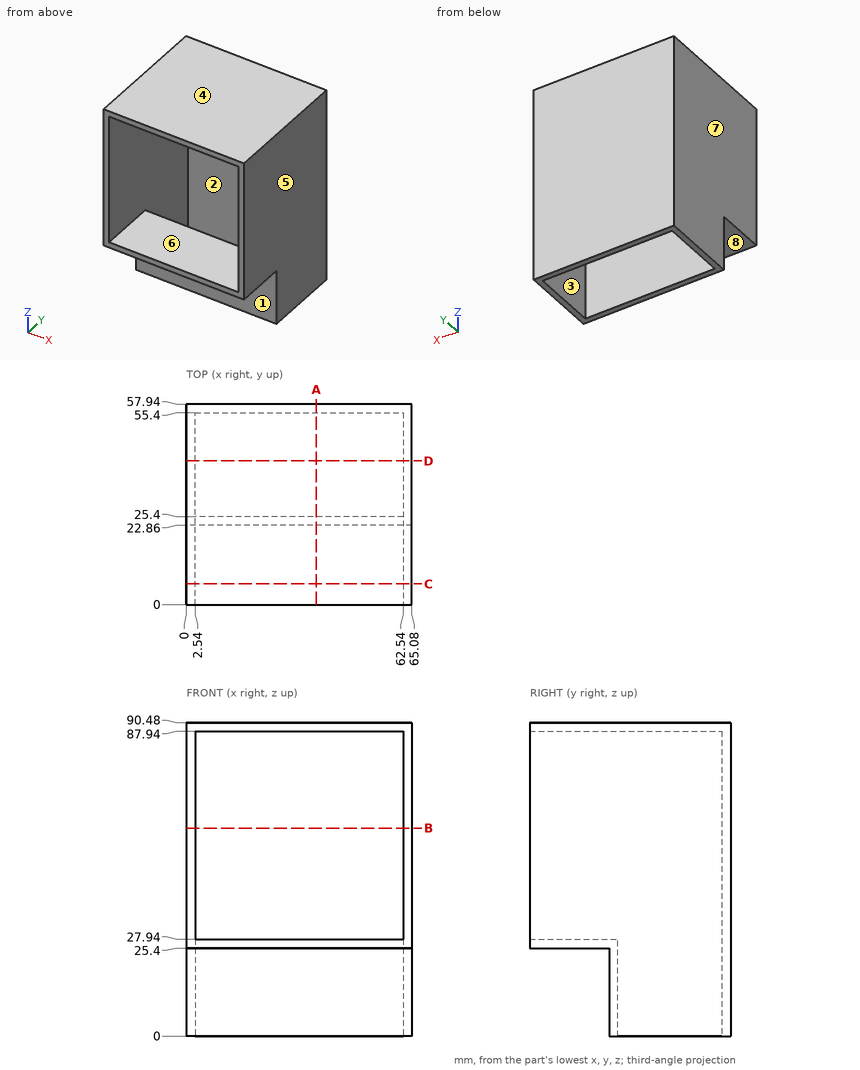
Job drawing, mm, ordinate dimensions from the low corner. One solid piece. A direction names the side the tool comes from. Coordinates: 2 decimals unless noted, no trailing zeros. Write each loop counter-clockwise with the first axis right and the second up, starting at its lowest first coordinate (ties: lowest second). Pieces come first, ordered by that corner, then holes. Notation, with made-up numbers: M -32,15.5 L 18,15.5 A24 ccw 18,49.5 Z; hole C 51.25,21 d6. An arc over 180 degrees is marked long. Answer as a JSON object with one key per item and string values. Group by question number.
1) Wall check: line 1 (X direction, y = 27, z = 41.5); line 2 (Y direction, x = 48.5, z = 5.5); line 3 (Z direction, x = 47.5, y = 8). Give the ranges that are in metal, low to high. Write a range as from..to.
2) Saw through at A-A (x = 37.5). Write the cut outline in (y, z), plus the area to 3 significant figures.
3) Saw through at C-C (y = 6). Write the cut outline in (x, z), plus the area to 3 significant figures.
4) Mould opens along X. For the marked faces 6, 7 and 8 say: +X half, -X half, draft (parallel to the pull), parting line (faces both ways), or undercut.
5) Saw through at B-B (z = 60). Write the cut outline in (x, y).
6) Saw through at D-D (y = 41.5). Write the cut outline in (x, z), plus the area to 3 significant figures.
7) Pin check, flat tips, straight feed: pin 1 Ø3 at (x, y) = (21, 36) entering from -Z; pin 2 Ø12.5 at (x, z) = (28, 7.5) entering from -Y; pin 3 Ø7 at (x, y) = (36, 9.5) entering from -Z; pin 4 Ø18 at (x, z) = (17.5, 23.5) entering from -Y. Stop position of each tip, or through.
8) Tool access for the marked faces 1, 2, 3, 4 and 5: list every direction of +Z, -Z, +X, -X, +Y, -Y with a clear straight run to the whole face (end or side of a thin tool).
Values follow:
{
 "1": {"line 1": "x = 0..2.54, 62.54..65.08", "line 2": "y = 22.86..25.4, 55.4..57.94", "line 3": "z = 25.4..27.94, 87.94..90.48"},
 "2": {"outline": "M 0,25.4 L 22.86,25.4 L 22.86,0 L 25.4,0 L 25.4,27.94 L 0,27.94 Z; M 0,87.94 L 55.4,87.94 L 55.4,0 L 57.94,0 L 57.94,90.48 L 0,90.48 Z", "area": "500 mm2"},
 "3": {"outline": "M 0,25.4 L 65.08,25.4 L 65.08,90.48 L 0,90.48 Z; hole M 2.54,27.94 L 62.54,27.94 L 62.54,87.94 L 2.54,87.94 Z", "area": "635 mm2"},
 "4": {"face 6": "undercut", "face 7": "-X half", "face 8": "draft"},
 "5": {"outline": "M 0,0 L 2.54,0 L 2.54,55.4 L 62.54,55.4 L 62.54,0 L 65.08,0 L 65.08,57.94 L 0,57.94 Z"},
 "6": {"outline": "M 0,0 L 2.54,0 L 2.54,87.94 L 62.54,87.94 L 62.54,0 L 65.08,0 L 65.08,90.48 L 0,90.48 Z", "area": "612 mm2"},
 "7": {"pin 1": "stops at z = 87.94", "pin 2": "stops at y = 22.86", "pin 3": "stops at z = 25.4", "pin 4": "stops at y = 0"},
 "8": {"face 1": "-Z, +X, -X, -Y", "face 2": "-Z", "face 3": "none", "face 4": "+Z, +X, -X, +Y, -Y", "face 5": "+Z, -Z, +X, +Y, -Y"}
}
